Verification items for the finished model (mm, model axes). Face numbers are marked on the shaded views. Coordinates: 2 decimals unless noted, no trailing zeros. Loops run counter-clockwise (first coordinate to the right, second up) from the corner with the lowest first, then second, coordinate; pieces in that order, holes last. Notation, with made-up numbers: (47, -14) -> (105, -14) arc R13 cw to (105, 10) -> close; hole circle Ø1 at (51.5, 81). An arc over 180 degrees is marked (long way). Answer as a JSON object with one key per item and string values. Group by question number.
Q1. Cross-section at A-A on x = -53.5. Record the boundary of the cut face in (y, z).
Q2. Release check for a two-part mould opening along Y. For the marked faces 1 and 2 record: released by +Y, released by -Y, zero draft, split by the parting line, or undercut.
Q3. Gauge pin test, flat ends, axial feed: pin 1 Ø1 at (x, z) = (0, -5) entering from +Y; pin 2 Ø6 at (x, z) = (15.5, 12) entering from +Y; pin 3 Ø1 at (y, z) = (-4.5, -9.5) entering from -X. Record the tip position at first contact, or that the pin passes through.
Q4. Scan lines: L1, parallel to X at y = 8.5, z = 3; L2, parallel to X at y = 11.75, z = -5.5; L3, parallel to Y at x = 46.5, z = -0.5. Record each from-to range of solid material in increasing order.
Autodesk Inventor part; units mm, degrees
ref_plane "YZ Plane" through (0, 0, 0) normal (1, 0, 0) x (0, 1, 0)
ref_plane "XZ Plane" through (0, 0, 0) normal (0, 1, 0) x (-1, 0, 0)
ref_plane "XY Plane" through (0, 0, 0) normal (0, 0, 1) x (1, 0, 0)
sketch "Sketch1" plane through (0, 0, 0) normal (0, 0, 1) x (1, 0, 0)
  line L0 (-82.5, 0) -> (82.5, 0)
  line L1 (-82.5, 0) -> (-82.5, 12.5)
  line L2 (-82.5, 12.5) -> (77.5, 12.5)
  line L3 (77.5, 12.5) -> (77.5, 15)
  line L4 (77.5, 15) -> (82.5, 15)
  line L5 (82.5, 15) -> (82.5, 0)
  circle A0 centre (-72.5, 0) radius 1.75
  line L6 (77.5, 12.75) -> (57.5, 12.5)
  line L7 (-82.5, 5) -> (-62.5, 5)
  line L8 (-62.5, 5) -> (-62.5, 12.5)
  point P0 (0, 0)
  point P1 (0, 0)
  dimension "d0" = 165
  dimension "d1" = 25
  dimension "d2" = 5
  dimension "d3" = 30
  dimension "d8" = 3.5
  dimension "d9" = 10
  dimension "d12" = 0.25
  dimension "d13" = 20
  dimension "d14" = 10
  dimension "d15" = 20
revolve "Revolution1" add sketch "Sketch1" angle 360 about axis through (-82.5, 0, 0) along (1, 0, 0) picked at (-71.9665, 0.4107) contours A0 L0 L1 L7 L8 L2 L3 L4 L5 | L0 A0 | L3 L2 L6
fillet "Fillet1" radius 1 1 edges at (-62.5, -5, 0)
thread "Thread1"
chamfer "Chamfer1" distance 1 angle 45 3 edges at (82.5, -15, 0) (-62.5, -12.5, 0) (-82.5, -5, 0)
properties part number "PWTR-0111" material "Stainless Steel"
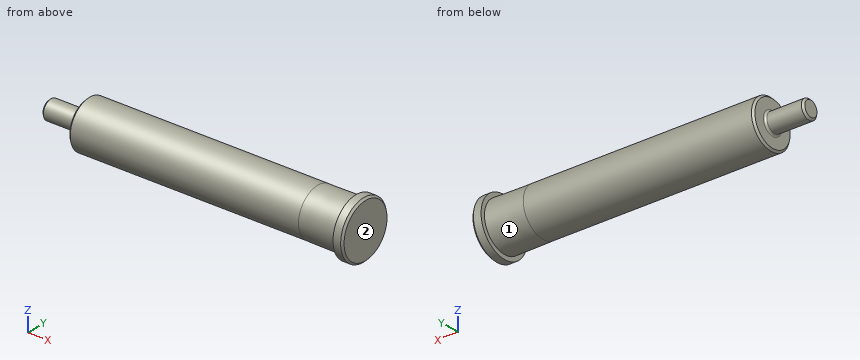
Computed values:
{
 "1": {"outline": "circle Ø25 at (0, 0)"},
 "2": {"face 1": "split by the parting line", "face 2": "zero draft"},
 "3": {"pin 1": "stops at y = 11.66", "pin 2": "stops at y = 8.67", "pin 3": "stops at x = -62.5"},
 "4": {"L1": "x = -62.5 to 82.5", "L2": "x = 77.5 to 82.5", "L3": "y = -12.49 to 12.49"}
}
